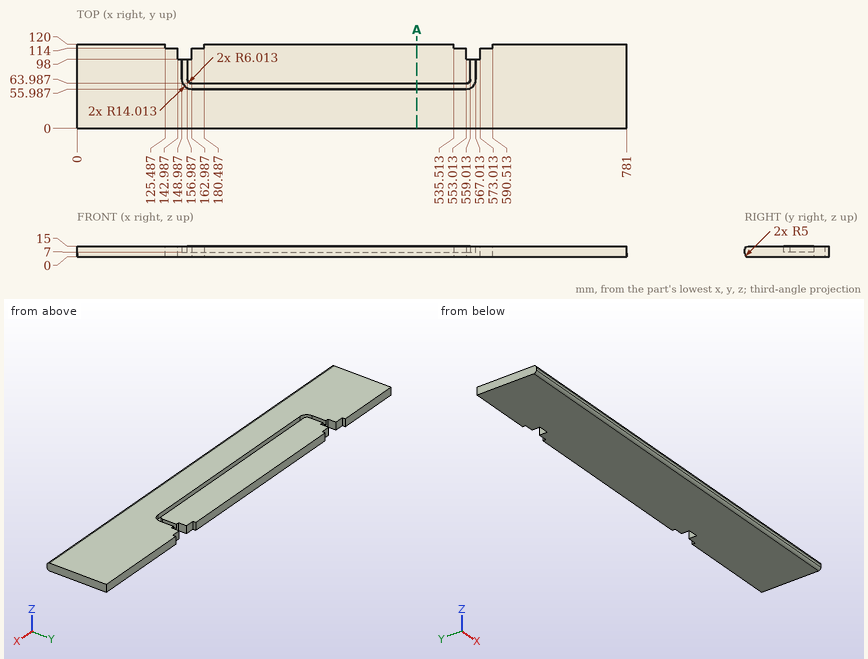
Design review of the part shown in the three views and the two pictorial views. Dimensions are in mm from the part's minimum x, y and z. Give positions to 0.01 mm unless a question says otherwise; leave off trailing zeros. Loops run counter-clockwise (first coordinate to the right, second up) from the corner with the lowest first, then second, coordinate; pieces in that order, holes last. Notation, with made-up numbers: (16, 84.5) -> (53, 84.5) arc R32 cw to (53, 119.5) -> close; hole circle Ø1 at (81, 89). An arc over 180 degrees is marked (long way). Answer as a JSON object with one key per item and string values. Group by question number.
Q1. Take a section at A-A (x = 483). Write out the cut boundary in (y, z).
Q2. Wall thickness on line 1 along X through (y, z) = (108, 13.5); line 2 along Y through (x, z) = (354, 10.5) (1 decimal); line 3 along X through (y, z) = (68, 7.25): over which ranges is each line inside the solid? List them lowest first.
Q3. Insertion check: pin 1 (7.5 mm diameter, centred on x = 148.5, z = 9.5, fed in from +Y); pin 2 (5 mm diameter, centred on y = 116, z = 9, fed in from -X); pin 3 (4.5 mm diameter, centred on x = 548, z = 9, fed in from +Y). Each pin has a flat end and moves straight along its axis. Give the tip position at first contact, or say it passes through.
Answer below:
{
 "1": {"outline": "(0, 5) arc R5 ccw to (5, 0) -> (120, 0) -> (120, 15) -> (63.99, 15) -> (63.99, 7) -> (55.99, 7) -> (55.99, 15) -> (5, 15) arc R5 ccw to (0, 10) -> close"},
 "2": {"line 1": "x = 0 to 142.99, 162.99 to 553.01, 573.01 to 781", "line 2": "y = 0 to 56, 64 to 120", "line 3": "x = 0 to 149.13, 157.33 to 558.67, 566.87 to 781"},
 "3": {"pin 1": "stops at y = 98", "pin 2": "stops at x = 0", "pin 3": "stops at y = 114"}
}
